Verification items for the finished model (mm, model axes). A direction names the side the tool comes from. Give positions to 0.01 mm unless a question says otherwise; leave off trailing zeros. Write each loop counter-clockwise with the first axis right and the second up, starting at its lowest first coordinate (ties: lowest second). Pieces come first, ordered by that corner, then holes. Notation, with made-up numbers: (-10, 55) -> (12, 55) arc R34 cw to (12, 91) -> close; hole circle Ø4 at (17, 51.25). An arc over 180 degrees is marked (long way). Answer as CSV lines item,"result". Start each with the question number.
1) Tool access check on faces 4 (the flat face through (3.503, 2.06, 1.628)), 5 (the flat face through (5.474, -3.219, 57.061)). Record the directions out of +Z, -Z, +X, -X, +Y, -Y that give a thin tool (end or side, any length) a straight path to the whole face; none if there is none.
2) Mould release check, pull along X, two halves, no side actions. Record for faces 1 (the flat face through (0, -6.35, 57)), 2 (the cylindrical face through (-0.64, 4.91, 24.42)), 3 (the flat face through (-1, 2, 3.302)): released by +X, released by -X, zero draft, split by the parting line, or undercut.
3) Sectioned sample at B-B on z = 20.5. Record the cut outline in (x, y).
4) Gauge pin test, flat ends, axial feed: pin 1 Ø3 at (x, z) = (1.5, 23) entering from -Y; pin 2 Ø4 at (y, z) = (-0.5, 44) entering from +X; pin 3 Ø1.7 at (x, z) = (-0.5, 1) entering from +Y. Record the tip position at first contact, or that the pin passes through.
5) Material ranges on L1, parallel to Y at x = 0, z = 25; L2, parallel to Z at x = 4.5, y = -0.25; L3, parallel to X at y = 1.75, z = 29, recorded low to high.
6) Sectioned sample at A-A on x = 0. Record the cut outline in (y, z), and give its area (3 significant figures).
7) Sectioned sample at C-C on z = 59.5. Record the cut outline in (x, y), and give its area (3 significant figures).
```python
from build123d import *

# Parameters (mm, degrees)
SKETCH2_R           = 4.953
SKETCH2_R_2         = 2.032
BOSS_EXTRUDE1_DEPTH = 50.8
CUT_EXTRUDE1_DEPTH  = 3.302
BOSS_EXTRUDE2_DEPTH = 12.7
FILLET1_R           = 1.27


with BuildPart() as part:
    # Sketch2 → Boss-Extrude1 (new body)
    with BuildSketch(Plane.XY):
        Circle(SKETCH2_R)
        Circle(SKETCH2_R_2, mode=Mode.SUBTRACT)
    extrude(amount=BOSS_EXTRUDE1_DEPTH)

    # Sketch3 → Cut-Extrude1 (cut)
    with BuildSketch(Plane(origin=(0, 0, 0), x_dir=(-1, 0, 0), z_dir=(0, 0, -1))):
        Polygon((4.692702988, 0), (2.346351494, 4.064), (-2.346351494, 4.064), (-4.692702988, 0), (-2.346351494, -4.064), (2.346351494, -4.064), align=None)
    extrude(amount=-CUT_EXTRUDE1_DEPTH, mode=Mode.SUBTRACT)

    # Sketch4 → Boss-Extrude2 (add)
    with BuildSketch(Plane.XY.offset(50.8)):
        Polygon((7.332348419, 0), (3.666174209, 6.35), (-3.666174209, 6.35), (-7.332348419, 0), (-3.666174209, -6.35), (3.666174209, -6.35), align=None)
    extrude(amount=BOSS_EXTRUDE2_DEPTH)

    # Fillet1
    fillet1_edges = [part.edges().sort_by_distance(p)[0] for p in [
        (-4.953, 0, 50.8),
    ]]
    fillet(fillet1_edges, radius=FILLET1_R)


solid = part.part
```
Ans:
1,face 4,"-Z"
1,face 5,"+Z, -Z, +X, -Y"
2,face 1,"zero draft"
2,face 2,"split by the parting line"
2,face 3,"undercut"
3,outline,"circle Ø9.91 at (0, 0); hole circle Ø4.06 at (0, 0)"
4,pin 1,"stops at y = -4.95"
4,pin 2,"stops at x = 4.95"
4,pin 3,"stops at y = 4.95"
5,L1,"y = -4.95 to -2.03, 2.03 to 4.95"
5,L2,"z = 3.3 to 63.5"
5,L3,"x = -4.63 to -1.03, 1.03 to 4.63"
6,outline,"(-6.35, 50.8) -> (-6.22, 50.8) arc R1.27 cw to (-4.95, 49.53) -> (-4.95, 0) -> (-4.06, 0) -> (-4.06, 3.3) -> (-2.03, 3.3) -> (-2.03, 50.8) -> (2.03, 50.8) -> (2.03, 3.3) -> (4.06, 3.3) -> (4.06, 0) -> (4.95, 0) -> (4.95, 49.53) arc R1.27 cw to (6.22, 50.8) -> (6.35, 50.8) -> (6.35, 63.5) -> (-6.35, 63.5) -> close"
6,area,"445 mm²"
7,outline,"(-7.33, 0) -> (-3.67, -6.35) -> (3.67, -6.35) -> (7.33, 0) -> (3.67, 6.35) -> (-3.67, 6.35) -> close"
7,area,"140 mm²"
